The model under review builds one solid part; all positions refer to its coordinate system, in mm. Round coordinates to 2 decimals unless told otherwise and drop trailing zeros. Order: outer loops, then holes, each group sorted by start corner. A loop starts at its lowest first (then second) coordinate and runs counter-clockwise, first axis right, second up. Notation, with made-up numbers: M 16,-24 L 60,-24 A32 ccw 60,2 Z; hole C -10,69 d6. An arc over 180 degrees is marked long. Use a Markdown table: item, result. Add a question column.
1. Consider section D-D on x = -4.5. State the section outline as (y, z) points.
2. To check wall thickness, follow probe 1 along Y at (x, z) = (0, 1.3); probe 2 along Y at (x, z) = (-1, 0.6); probe 3 along X at (y, z) = (22.5, 0.5). State the ranges of each line that lie inside material, in increasing order.
3. Consider section A-A on x = 0. State the section outline as (y, z) points.
4. The part is to be moulded in two halves that separate along Y. For faces 1 (the flat face through (0, 14, 0)), 2 (the flat face through (7.462, 11.228, 0.74)), 3 (the cylindrical face through (-0.716, 18.547, 0.74)), say which applies: +Y half, -Y half, draft (parallel to the pull), parting line (faces both ways), or undercut.
5. Consider section B-B on y = 24. State the section outline as (x, z) points.
6. Consider section C-C on z = 0.75. State the section outline as (x, y) points (3 decimals), then the cut area to 3 significant figures.
Autodesk Inventor part; units mm, degrees
ref_plane "YZ Plane" through (0, 0, 0) normal (1, 0, 0) x (0, 1, 0)
ref_plane "XZ Plane" through (0, 0, 0) normal (0, 1, 0) x (-1, 0, 0)
ref_plane "XY Plane" through (0, 0, 0) normal (0, 0, 1) x (1, 0, 0)
sketch "Sketch1" plane through (0, 0, 0) normal (0, 0, 1) x (1, 0, 0)
  circle A0 centre (0, 0) radius 1.45
  line L0 (0, 0) -> (-32, 0) construction
  arc A1 (-6, 0) -> (5.9529, -0.75) centre (0, 0) ccw
  circle A2 centre (0, 24) radius 5.5
  arc A3 (8.9294, 22.875) -> (-8.9294, 22.875) centre (0, 24) ccw
  line L1 (8.9294, 22.875) -> (5.9529, -0.75)
  line L2 (-5.9529, -0.75) -> (-8.9294, 22.875)
  dimension "d0" = 2.9
  dimension "d61" = 6
  dimension "d63" = 24
  dimension "d69" = 9
  dimension "d72" = 11
extrude "Extrusion1" add sketch "Sketch1" along normal blind 1.5
properties part number "tipper_link_B_support"
Answer block:
| question | item | result |
|---|---|---|
| 1 | outline | M -3.97,0 L 20.84,0 L 20.84,1.5 L -3.97,1.5 Z; M 27.16,0 L 31.79,0 L 31.79,1.5 L 27.16,1.5 Z |
| 2 | probe 1 | -6 to -1.45, 1.45 to 18.5, 29.5 to 33 |
| 2 | probe 2 | -5.92 to -1.05, 1.05 to 18.59, 29.41 to 32.94 |
| 2 | probe 3 | -8.88 to -5.29, 5.29 to 8.88 |
| 3 | outline | M -6,0 L -1.45,0 L -1.45,1.5 L -6,1.5 Z; M 1.45,0 L 18.5,0 L 18.5,1.5 L 1.45,1.5 Z; M 29.5,0 L 33,0 L 33,1.5 L 29.5,1.5 Z |
| 4 | face 1 | draft |
| 4 | face 2 | -Y half |
| 4 | face 3 | undercut |
| 5 | outline | M -9,0 L -5.5,0 L -5.5,1.5 L -9,1.5 Z; M 5.5,0 L 9,0 L 9,1.5 L 5.5,1.5 Z |
| 6 | outline | M -8.929,22.875 L -5.953,-0.75 A6 ccw 5.953,-0.75 L 8.929,22.875 A9 ccw long Z; hole C 0,24 d11; hole C 0,0 d2.9 |
| 6 | area | 445 mm^2 |
